Model file for the job. Use its own axes, mm. A direction names the side the tool comes from. Give positions to 0.01 mm unless a question says otherwise; leave off trailing zeros. Write each loop counter-clockwise with the first axis right and the second up, starting at its lowest first coordinate (ties: lowest second). Pieces come first, ordered by that corner, then holes. Notation, with made-up numbers: (-1.75, -1) - (52.25, -1) arc R25 ccw to (52.25, 33) - close; hole circle Ø2 at (55, 7). An arc over 180 degrees is marked (long way). One line per item, written item: value. Start each with the question number.
(1) Probe L1, parallel to Y at x = 75.5, z = 7; L2, parallel to Y at x = 17.5, z = 5.5; L3, parallel to X at y = 22.5, z = 4.5. List the from-to ranges inside material, lowest first.
(2) 3-axis set-ups, long thin cutter, end or side, ignore diameter. For faces 1 (the face through (39.92, 8.54, 5.75)), 2 (the face through (14.79, 6.297, 4.56)): which of +Z, -Z, +X, -X, +Y, -Y reach the whole face in a straight line?
(3) Cut at A-A, the plane x = 58. List the corners of the cut face in (y, z), and give its area (3 significant figures).
(4) Mould opens along X. For faces 3 (the face through (75, 37, 5)), 4 (the face through (5.26, 32.01, 4.56)), 5 (the face through (78.92, 14.59, 5.75)), 6 (the face through (135, 18, 5)) say: pulls with the +X half, pulls with the -X half, needs draft (parallel to the pull), parting line crosses it, or undercut.
(5) Drop flat-ended pins along their axis: P1, Ø4, axis at y = 10.5, z = 5.5, coming from the -X side; P2, Ø2, axis at y = 14, z = 5.5, coming from the -X side. Give the stop position or say it passes through.
from build123d import *

# Parameters (mm, degrees)
F0_R     = 12.5
F1_DEPTH = 9.25


with BuildPart() as f1:
    # F0 (on Top) → F1 (new body)
    with BuildSketch(Plane.XY):
        with BuildLine():
            ThreePointArc((0, 17.5), (5.125631, 5.125631), (17.5, 0))
            Line((17.5, 0), (130, 0))
            ThreePointArc((130, 0), (133.535534, 1.464466), (135, 5))
            Line((135, 5), (135, 32))
            ThreePointArc((135, 32), (133.535534, 35.535534), (130, 37))
            Line((130, 37), (17.5, 37))
            ThreePointArc((17.5, 37), (5.125631, 31.874369), (0, 19.5))
            Line((0, 19.5), (0, 17.5))
        make_face()
        with Locations((17.5, 18.5)):
            Circle(F0_R, mode=Mode.SUBTRACT)
    extrude(amount=F1_DEPTH)

    # F2 (on face) → F3 (revolve, cut)
    with BuildSketch(Plane.XY.offset(9.25)):
        Polygon((45, 35), (40, 35), (40, 33), (40, 13), (40, 2), (43, 2), (43.5, 6), (43.5, 11), (44.5, 14), (43.5, 14), (43.5, 33), (45, 33), align=None)
    revolve(axis=Axis((40, 23, 9.25), (0, -1, 0)), mode=Mode.SUBTRACT)

    # F2 (on face) → F4 (revolve, cut)
    with BuildSketch(Plane.XY.offset(9.25)):
        Polygon((64.5, 29), (58, 29), (58, 25), (58, 21), (58, 8), (61.5, 8), (61.5, 21), (66, 21), (66, 25), (64.5, 25), align=None)
    revolve(axis=Axis((58, 14.5, 9.25), (0, -1, 0)), mode=Mode.SUBTRACT)

    # F2 (on face) → F5 (revolve, cut)
    with BuildSketch(Plane.XY.offset(9.25)):
        Polygon((85.5, 29), (79, 29), (79, 25), (79, 21), (79, 8), (82.5, 8), (82.5, 21), (87, 21), (87, 25), (85.5, 25), align=None)
    revolve(axis=Axis((79, 14.5, 9.25), (0, -1, 0)), mode=Mode.SUBTRACT)

    # F2 (on face) → F6 (revolve, cut)
    with BuildSketch(Plane.XY.offset(9.25)):
        Polygon((106.5, 29), (100, 29), (100, 25), (100, 21), (100, 8), (103.5, 8), (103.5, 21), (108, 21), (108, 25), (106.5, 25), align=None)
    revolve(axis=Axis((100, 14.5, 9.25), (0, -1, 0)), mode=Mode.SUBTRACT)

    # F2 (on face) → F7 (revolve, cut)
    with BuildSketch(Plane.XY.offset(9.25)):
        Polygon((127.5, 29), (121, 29), (121, 25), (121, 21), (121, 8), (124.5, 8), (124.5, 21), (129, 21), (129, 25), (127.5, 25), align=None)
    revolve(axis=Axis((121, 14.5, 9.25), (0, -1, 0)), mode=Mode.SUBTRACT)


solid = f1.part
Answers follow:
1. L1: y = 0 to 21, 29 to 37
1. L2: y = 0 to 6, 31 to 37
1. L3: x = 0.26 to 5.66, 29.34 to 51.56, 64.44 to 72.56, 85.44 to 93.56, 106.44 to 114.56, 127.44 to 135
2. face 1: +Z
2. face 2: +Z, -Z
3. outline: (0, 0) - (37, 0) - (37, 9.25) - (29, 9.25) - (29, 2.75) - (25, 2.75) - (25, 1.25) - (21, 1.25) - (21, 5.75) - (8, 5.75) - (8, 9.25) - (0, 9.25) - close
3. area: 239 mm²
4. face 3: needs draft
4. face 4: pulls with the -X half
4. face 5: undercut
4. face 6: pulls with the +X half
5. P1: stops at x = 0.73
5. P2: stops at x = 0.18
